Input: part model. Units: mm. Frame: model coordinates. A direction names the side the tool comes from. Round coordinates to 2 decimals unless told otherwise and drop trailing zeros. Loops run counter-clockwise (first coordinate to the right, second up) from the corner with the lowest first, then second, coordinate; pieces in that order, holes last. Notation, with made-up numbers: (-7, -0.75) -> (44, -0.75) arc R7 cw to (44, 3.25) -> close; hole circle Ø2 at (10.25, 87). An arc over 180 degrees is marked (long way). Answer as a JSON object with one key per item and string values. Group by question number.
Item 1: Set-up query: faces 1 (the flat face through (0, -13, 30)), 2 (the flat face through (-3.8, -13, 50)), 3 (the flat face through (3.8, -14, 50)), 4 (the flat face through (0, -51.179, 49)). Return all of +Z, -Z, +X, -X, +Y, -Y with unobstructed straight access to the full face (end or side cutting, diameter ignored); none if empty.
Item 2: Section query A-A on x = 0. Return loops of the section in (y, z), and give its area (3 significant figures).
Item 3: Pin query (flat end, axial travel): pin 1 (20 mm diameter, centred on y = -29, z = 47.5, fed in from +X); pin 2 (4 mm diameter, centred on x = 1.5, z = 81, fed in from +Y); pin 3 (20 mm diameter, centred on y = -13, z = 53.5, fed in from -X). Return the tip coordinate at first contact, or that it passes through.
Item 4: Material intervals for line 1 (Z direction, x = -0.5, y = -40); line 2 (X direction, y = -50, z = 90); line 3 (Y direction, x = -0.5, z = 85), sorted ascending. Write a range as [from, to].
Item 5: Draft query along X for faces 5 (the cylindrical face through (-4.671, -50.734, 49.3)), 6 (the flat face through (0, -14, 70)), 7 (the cylindrical face through (1.2, -49.7, 11.6)). Return one class per face: released by +X, released by -X, zero draft, split by the parting line, or undercut.
Item 6: Section query C-C on y = 7.5. Return loops of the section in (x, z), and give its area (3 significant figures).
Item 7: Section query D-D on z = 65. Return loops of the section in (x, y), and give its area (3 significant figures).
Item 8: Section query B-B on z = 10. Return loops of the section in (x, y).
from build123d import *

# Parameters (mm, degrees)
RESSALTO_EXTRUS_O2_DEPTH   = 100
CORTE_EXTRUS_O4_DEPTH      = 30
CORTE_EXTRUS_O4_DEPTH_BACK = 1
ESBO_O2_W                  = 7.6
ESBO_O2_H                  = 70
CORTE_EXTRUS_O5_DEPTH      = 30
CORTE_EXTRUS_O7_DEPTH      = 21
CORTE_EXTRUS_O7_DEPTH_BACK = 22
F_3DSKETCH4_R              = 2
CORTE_EXTRUS_O8_START      = -3.8
CORTE_EXTRUS_O8_OUTLINE_R  = 4
CORTE_EXTRUS_O8_DEPTH      = 7.6


# Read off the part's stored shape, not the designer's step: Corte-extrusão8
with BuildPart() as part:
    # Esboço1 → Ressalto-extrusão2 (new body)
    with BuildSketch(Plane.XY):
        with BuildLine():
            Line((-3.8, -48.178624659), (-5.7, -48.178624659))
            Line((-5.7, -48.178624659), (-5.360626179, -49.63308389))
            ThreePointArc((-5.360626179, -49.63308389), (-4.656141559, -50.745296045), (-3.41294376, -51.178624659))
            Line((-3.41294376, -51.178624659), (3.41294376, -51.178624659))
            ThreePointArc((3.41294376, -51.178624659), (4.656141559, -50.745296045), (5.360626179, -49.63308389))
            Line((5.360626179, -49.63308389), (5.7, -48.178624659))
            Line((5.7, -48.178624659), (3.8, -48.178624659))
            Line((3.8, -48.178624659), (3.8, 21.821375341))
            Line((3.8, 21.821375341), (-3.8, 21.821375341))
            Line((-3.8, 21.821375341), (-3.8, -48.178624659))
        make_face()
    extrude(amount=RESSALTO_EXTRUS_O2_DEPTH)

    # Esboço2 → Corte-extrusão4 (cut, two sides: drawn at the far end of the back side and taken through both)
    with BuildSketch(Plane.XY.offset(-CORTE_EXTRUS_O4_DEPTH_BACK)):
        with Locations((0, -13.178624659)):
            Rectangle(ESBO_O2_W, ESBO_O2_H)
    extrude(amount=CORTE_EXTRUS_O4_DEPTH + CORTE_EXTRUS_O4_DEPTH_BACK, mode=Mode.SUBTRACT)

    # 3DSketch1 → Corte-extrusão5 (cut)
    with BuildSketch(Plane(origin=(-3.8, 21.821375341, 100), x_dir=(0.10793712415834626, -0.9941577225110841, 0), z_dir=(0, 0, 1))):
        Polygon((0, 0), (0.820322144, 7.555598691), (70.411362719, 0), (69.591040576, -7.555598691), align=None)
    extrude(amount=-CORTE_EXTRUS_O5_DEPTH, mode=Mode.SUBTRACT)

    # 3DSketch4 → Corte-extrusão7 (cut, two sides: drawn at the far end of the back side and taken through both)
    with BuildSketch(Plane(origin=(0, -48.178624659, 10), x_dir=(0, 0, 1), z_dir=(0, 1, 0)).offset(-CORTE_EXTRUS_O7_DEPTH_BACK)):
        with Locations(Location((0, 0, 0), (0, 0, 180))):
            Circle(F_3DSKETCH4_R)
        with Locations(Location((80, 0, 0), (0, 0, 180))):
            Circle(F_3DSKETCH4_R)
    extrude(amount=CORTE_EXTRUS_O7_DEPTH + CORTE_EXTRUS_O7_DEPTH_BACK, mode=Mode.SUBTRACT)

    # Corte-extrusão8 outline → Corte-extrusão8 (cut)
    with BuildSketch(Plane.YZ.offset(CORTE_EXTRUS_O8_START)):
        with Locations((5.45168837, 50)):
            Circle(CORTE_EXTRUS_O8_OUTLINE_R)
    extrude(amount=CORTE_EXTRUS_O8_DEPTH, mode=Mode.SUBTRACT)


solid = part.part
Solved:
{
 "1": {"face 1": "-Z, +X, -X, +Y", "face 2": "+Z, -Z, -X, +Y", "face 3": "+Z, -Z, +X, +Y", "face 4": "+Z, -Z, +X, -X, -Y"},
 "2": {"outline": "(-51.18, 0) -> (-48.18, 0) -> (-48.18, 8) -> (-51.18, 8) -> close; (-51.18, 12) -> (-48.18, 12) -> (-48.18, 30) -> (21.82, 30) -> (21.82, 70) -> (-48.18, 70) -> (-48.18, 88) -> (-51.18, 88) -> close; (-51.18, 92) -> (-48.18, 92) -> (-48.18, 100) -> (-51.18, 100) -> close; hole circle Ø8 at (5.45, 50)", "area": "3,030 mm²"},
 "3": {"pin 1": "x = 3.8", "pin 2": "y = -48.18", "pin 3": "x = -3.8"},
 "4": {"line 1": "[30, 70]", "line 2": "[-5.24, -2], [2, 5.24]", "line 3": "[-51.18, -48.18]"},
 "5": {"face 5": "released by -X", "face 6": "zero draft", "face 7": "undercut"},
 "6": {"outline": "(-3.8, 30) -> (3.8, 30) -> (3.8, 46.56) -> (-3.8, 46.56) -> close; (-3.8, 53.44) -> (3.8, 53.44) -> (3.8, 70) -> (-3.8, 70) -> close", "area": "252 mm²"},
 "7": {"outline": "(-5.7, -48.18) -> (-5.36, -49.63) arc R2 ccw to (-3.41, -51.18) -> (3.41, -51.18) arc R2 ccw to (5.36, -49.63) -> (5.7, -48.18) -> (3.8, -48.18) -> (3.8, 21.82) -> (-3.8, 21.82) -> (-3.8, -48.18) -> close", "area": "563 mm²"},
 "8": {"outline": "(-5.7, -48.18) -> (-5.36, -49.63) arc R2 ccw to (-3.41, -51.18) -> (-2, -51.18) -> (-2, -48.18) -> close; (2, -51.18) -> (3.41, -51.18) arc R2 ccw to (5.36, -49.63) -> (5.7, -48.18) -> (2, -48.18) -> close"}
}
